```python
from build123d import *

# Parameters (mm, degrees)
F0_W     = 152.4
F0_H     = 76.2
F1_DEPTH = 9.525
F2_W     = 9.525
F2_H     = 76.2
F3_DEPTH = 28.575
F5_D     = 6.5278


with BuildPart() as f1:
    # F0 (on Front) → F1 (new body)
    with BuildSketch(Plane.XZ):
        with Locations((76.2, 38.1)):
            Rectangle(F0_W, F0_H)
        with BuildLine():
            ThreePointArc((135.724848, 48.909018), (130.42042, 27.634117), (122.206719, 7.304495))
            ThreePointArc((122.206719, 7.304495), (115.83847, 5.111731), (113.645706, 11.47998))
            ThreePointArc((113.645706, 11.47998), (121.361606, 30.577503), (126.344555, 50.563017))
            ThreePointArc((126.344555, 50.563017), (131.861701, 54.426165), (135.724848, 48.909018))
        make_face(mode=Mode.SUBTRACT)
    extrude(amount=F1_DEPTH)

    # F2 (on face) → F3 (join)
    with BuildSketch(Plane.XZ.offset(9.525)):
        with Locations((4.7625, 38.1)):
            Rectangle(F2_W, F2_H)
    extrude(amount=F3_DEPTH)

    # F5 (through all)
    with Locations(Plane(origin=(0, 0, 0), x_dir=(0, -1, 0), z_dir=(-1, 0, 0))):
        with Locations((19.05, 69.85), (19.05, 6.35)):
            Hole(F5_D / 2)


solid = f1.part
```
Design review of the part built by this model. Coordinates are the model's own, in mm. A direction names the side the tool comes from. Give positions to 0.01 mm unless a question says otherwise; leave off trailing zeros. Write each loop counter-clockwise with the first axis right and the second up, starting at its lowest first coordinate (ties: lowest second). Pieces come first, ordered by that corner, then holes. Notation, with made-up numbers: (-10.5, 64) - (2.5, 64) arc R14 cw to (2.5, 76) - close; hole circle Ø5 at (10.5, 61). An arc over 180 degrees is marked (long way). Return JSON: item names as keys, results as strings. Group by question number.
(1) We need section C-C, the plane z = 57. Give the boundary of the cut face in (x, y) (3 decimals), then the cut area to 3 significant figures.
(2) Machinability: for faces 1 (the flat face through (9.525, -24, 38)), 2 (the flat face through (75, 0, 39)), 3 (the cylindrical face through (131.758, -4.696, 54.443)), which of the approach directions +Z, -Z, +X, -X, +Y, -Y give a long, thin tool a straight path to every point of the face, cutting with its end or side? Answer none if there is none.
(3) Mouldability with a two-part tool opening along Z and no side actions: class faces 4 (the cylindrical face through (130.515, -4.696, 27.926)), 5 (the flat face through (0, -19, 38)), 6 (the cylindrical face through (4.829, -19.758, 66.664)), 7 (the flat face through (65, -9, 76.2)) as +Z half, -Z half, draft (parallel to the pull), parting line (faces both ways), or undercut.
(4) We need section B-B, the plane y = -19.05. Give the boundary of the cut face in (x, z) (3 decimals).
(5) Insertion check: pin 1 (1 mm diameter, centred on x = 78, z = 47.5, fed in from -Y) (3 decimals); pin 2 (4 mm diameter, centred on y = -19.05, z = 6.35, fed in from -X); pin 3 (14.5 mm diameter, centred on y = -29.5, z = 33.5, fed in from +X) (3 decimals). Each pin has a flat end and moves straight along its axis. Give the tip position at first contact, or say it passes through.
(6) We need section A-A, the plane z = 69.85. Give the boundary of the cut face in (x, y) (3 decimals), then the cut area to 3 significant figures.
(7) To check wall thickness, follow probe 1 along Z at (x, y) = (6.75, -19.05); probe 2 along X at (y, z) = (-29, 6) (3 decimals); probe 3 along X at (y, z) = (-7.5, 35.5). State the ranges of each line that lie inside material, in increasing order.
(8) We need section D-D, the plane x = 67.5. Give the boundary of the cut face in (y, z) (3 decimals).
Reported:
{
 "1": {"outline": "(0, -38.1) - (9.525, -38.1) - (9.525, -9.525) - (152.4, -9.525) - (152.4, 0) - (0, 0) - close", "area": "1,720 mm2"},
 "2": {"face 1": "+Z, -Z, +X, -Y", "face 2": "+Z, -Z, +X, -X, +Y", "face 3": "+Y, -Y"},
 "3": {"face 4": "undercut", "face 5": "draft", "face 6": "undercut", "face 7": "+Z half"},
 "4": {"outline": "(0, 0) - (9.525, 0) - (9.525, 3.086) - (0, 3.086) - close; (0, 9.614) - (9.525, 9.614) - (9.525, 66.586) - (0, 66.586) - close; (0, 73.114) - (9.525, 73.114) - (9.525, 76.2) - (0, 76.2) - close"},
 "5": {"pin 1": "stops at y = -9.525", "pin 2": "passes through", "pin 3": "stops at x = 9.525"},
 "6": {"outline": "(0, -38.1) - (9.525, -38.1) - (9.525, -22.314) - (0, -22.314) - close; (0, -15.786) - (9.525, -15.786) - (9.525, -9.525) - (152.4, -9.525) - (152.4, 0) - (0, 0) - close", "area": "1,660 mm2"},
 "7": {"probe 1": "z = 0 to 3.09, 9.61 to 66.59, 73.11 to 76.2", "probe 2": "x = 0 to 9.525", "probe 3": "x = 0 to 122.87, 132.75 to 152.4"},
 "8": {"outline": "(-9.525, 0) - (0, 0) - (0, 76.2) - (-9.525, 76.2) - close"}
}
